```python
from build123d import *

# Parameters (mm, degrees)
BOSS_EXTRUDE1_DEPTH = 114.3
CUT_EXTRUDE2_DEPTH  = 17.78
LPATTERN2_COUNT     = 3
LPATTERN2_PITCH     = 46.99
SKETCH5_W           = 26.67
SKETCH5_H           = 35.56
CUT_EXTRUDE3_DEPTH  = 5.334
SKETCH6_W           = 2.54
SKETCH6_H           = 4.826
SKETCH6_W_2         = 29.21
CUT_EXTRUDE4_DEPTH  = 7.35
CHAMFER1_SIZE       = 1.016


with BuildPart() as part:
    # Sketch2 → Boss-Extrude1 (new body)
    with BuildSketch(Plane(origin=(0, 0, 0), x_dir=(0, 0, -1), z_dir=(1, 0, 0))):
        Polygon((0, -19.05), (-3.175, -23.876), (3.175, -23.876), (3.175, -19.05), (3.175, 19.05), (-3.175, 19.05), (-3.175, -19.05), align=None)
    extrude(amount=BOSS_EXTRUDE1_DEPTH)

    # Sketch4 → Cut-Extrude2 (cut)
    with BuildSketch(Plane(origin=(114.3, 0, 0), x_dir=(0, 0, -1), z_dir=(1, 0, 0))):
        Polygon((-3.175, 14.732), (-3.175, 11.277980125), (1.778, 8.019427494), (1.778, 14.732), align=None)
        Polygon((-3.175, 3.429), (-3.175, -0.304039749), (1.905, -3.646145012), (1.905, 3.429), align=None)
        Polygon((-3.175, -7.874), (2.032, -7.874), (2.032, -15.311717518), (-3.175, -11.886059624), align=None)
    cut_extrude2 = extrude(amount=-CUT_EXTRUDE2_DEPTH, mode=Mode.SUBTRACT)

    # LPattern2: Cut-Extrude2 ×3
    with Locations(*[(-i * LPATTERN2_PITCH, 0, 0) for i in range(1, LPATTERN2_COUNT)]):
        add(cut_extrude2, mode=Mode.SUBTRACT)

    # Sketch5 → Cut-Extrude3 (cut)
    with BuildSketch(Plane.XY.offset(3.175)):
        with Locations((80.645, 0)):
            Rectangle(SKETCH5_W, SKETCH5_H)
        with Locations((33.655, 0)):
            Rectangle(SKETCH5_W, SKETCH5_H)
    extrude(amount=-CUT_EXTRUDE3_DEPTH, mode=Mode.SUBTRACT)

    # Sketch6 → Cut-Extrude4 (cut, through all)
    with BuildSketch(Plane.XY.offset(3.175)):
        with Locations((1.27, -21.463)):
            Rectangle(SKETCH6_W, SKETCH6_H)
        with Locations((34.925, -21.463)):
            Rectangle(SKETCH6_W_2, SKETCH6_H)
        with Locations((81.915, -21.463)):
            Rectangle(SKETCH6_W_2, SKETCH6_H)
    extrude(amount=-CUT_EXTRUDE4_DEPTH, mode=Mode.SUBTRACT)

    # Chamfer1
    chamfer1_edges = [part.edges().sort_by_distance(p)[0] for p in [
        (2.54, -21.463, 1.5875),
        (2.54, -21.463, -3.175),
        (2.54, -23.876, 0),
        (49.53, -21.463, 1.5875),
        (49.53, -21.463, -3.175),
        (49.53, -23.876, 0),
        (96.52, -21.463, 1.5875),
        (96.52, -21.463, -3.175),
        (96.52, -23.876, 0),
    ]]
    chamfer(chamfer1_edges, length=CHAMFER1_SIZE)


solid = part.part
```
Here's how the part is built. I have some questions about the finished solid (model axes, mm). A direction names the side the tool comes from. Coordinates: 2 decimals unless noted, no trailing zeros. Order: outer loops, then holes, each group sorted by start corner. A loop starts at its lowest first (then second) coordinate and runs counter-clockwise, first axis right, second up. Notation, with made-up numbers: (-10, 18.5) - (26, 18.5) arc R22 cw to (26, 52.5) - close; hole circle Ø8 at (61.5, 80). An arc over 180 degrees is marked (long way). One line per question, with ' | ' between items.
(1) Suppose I cut it at D-D on x = 18. List the corners of the cut face in (y, z) for me (3 decimals), and give its area (3 significant figures).
Report:
outline: (-23.876, -3.175) - (19.05, -3.175) - (19.05, 3.175) - (14.732, 3.175) - (14.732, -1.778) - (8.019, -1.778) - (11.278, 3.175) - (3.429, 3.175) - (3.429, -1.905) - (-3.646, -1.905) - (-0.304, 3.175) - (-7.874, 3.175) - (-7.874, -2.032) - (-15.312, -2.032) - (-11.886, 3.175) - (-19.05, 3.175) - (-19.05, 0) - (-23.876, 3.175) - close | area: 182 mm2
(2) Suppose I cut it at B-B on x = 84.5. List the corners of the cut face in (y, z) for me (3 decimals).
Report:
outline: (-19.05, -3.175) - (19.05, -3.175) - (19.05, 3.175) - (17.78, 3.175) - (17.78, -2.159) - (-17.78, -2.159) - (-17.78, 3.175) - (-19.05, 3.175) - close
(3) For faces 5 (the flat face through (2.54, -21, -1)), 6 (the flat face through (59, 0, -1.905)), 7 (the flat face through (20.32, -21, -1)), 8 (the flat face through (106, 0, -1.905)), 9 (the flat face through (59, 3.429, 1)), which set-ups out of +Z, -Z, +X, -X, +Y, -Y let a thin tool reach every point of the face, with its end or its side?
Report:
face 5: +Z, -Z, -X, -Y | face 6: none | face 7: +Z, -Z, -Y | face 8: +X | face 9: +Z
(4) Suppose I cut it at C-C on y = -16.5. List the corners of the cut face in (x, z) for me (3 decimals), and give its area (3 significant figures).
Report:
outline: (0, -3.175) - (114.3, -3.175) - (114.3, 3.175) - (93.98, 3.175) - (93.98, -2.159) - (67.31, -2.159) - (67.31, 3.175) - (46.99, 3.175) - (46.99, -2.159) - (20.32, -2.159) - (20.32, 3.175) - (0, 3.175) - close | area: 441 mm2
(5) Will these pins go through, and if not, where does the flat tip stop? pin 1 (8 mm diameter, centred on x = 56.5, y = 0.5, fed in from +Z) (3 decimals); pin 2 (2 mm diameter, centred on x = 57.5, y = -10.5, fed in from +Z).
Report:
pin 1: stops at z = 3.175 | pin 2: stops at z = -2.03
(6) Suppose I cut it at A-A on y = 1. List the corners of the cut face in (x, z) for me (3 decimals).
Report:
outline: (0, -3.175) - (114.3, -3.175) - (114.3, -1.905) - (96.52, -1.905) - (96.52, 3.175) - (93.98, 3.175) - (93.98, -2.159) - (67.31, -2.159) - (67.31, -1.905) - (49.53, -1.905) - (49.53, 3.175) - (46.99, 3.175) - (46.99, -2.159) - (20.32, -2.159) - (20.32, -1.905) - (2.54, -1.905) - (2.54, 3.175) - (0, 3.175) - close
(7) If we mould it in two halves opening along Z, with no side actions, what happens to faces 1 (the flat face through (12, -12, -2.032)), 2 (the flat face through (11.821, -21.429, 1.565)), 3 (the flat face through (96.52, 1, 1)), 4 (the flat face through (59, 14.732, 1))? For each: pulls with the +Z half, pulls with the -Z half, needs draft (parallel to the pull), parting line crosses it, or undercut.
Report:
face 1: undercut | face 2: pulls with the +Z half | face 3: undercut | face 4: needs draft
(8) If I drill on L1, parallel to X at y = 17, z = 2.75; L2, parallel to X at y = -1.5, z = -1; L3, parallel to Y at x = 88.5, z = -2, over which ranges is the centre line in solid material (lowest first)?
Report:
L1: x = 0 to 20.32, 46.99 to 67.31, 93.98 to 114.3 | L2: x = 0 to 2.54, 46.99 to 49.53, 93.98 to 96.52 | L3: y = -19.05 to -17.78, 17.78 to 19.05
